Part print with two shaded views. Sizes in mm from the minimum x, y, z corner. A direction names the side the tool comes from. Round coordinates to 2 decimals unless told otherwise and drop trailing zeros. Order: outer loops, then holes, each group sorted by start corner. A loop starts at its lowest first (then second) coordinate and runs counter-clockwise, first axis right, second up. Notation, with made-up numbers: (28, 48) -> (56, 48) arc R14 cw to (56, 56) -> close; hole circle Ø9 at (-20.75, 24.25). An arc over 180 degrees is marked (long way). Use a Markdown table: item, result. Add a question column.
Item 1: Slice it at A-A, the plane z = 1.75. Give the cut face in (x, y) (3 decimals).
Item 2: 3-axis set-ups, long thin cutter, end or side, ignore diameter. For the marked faces 1, 2, 3, 4 and 5: which of +Z, -Z, +X, -X, +Y, -Y reach the whole face in a straight line?
Item 3: Slice it at C-C, the plane y = 9.5. Give the cut face in (x, z) (3 decimals), plus the area to 3 significant figures.
Item 4: Two-plate mould, pull along X, no slides. Class the marked faces 6, 7 and 8: released by +X, released by -X, zero draft, split by the parting line, or undercut.
Item 5: Probe L1, parallel to Z at x = 2.25, y = 20 (3 decimals); L2, parallel to Y at x = 8.75, z = 5 (3 decimals); L3, parallel to Y at x = 13, z = 3. List the from-to ranges inside material, lowest first.
Item 6: Slice it at D-D, the plane z = 3.75. Give the cut face in (x, y) (3 decimals).
Item 7: Pin check, flat tips, straight feed: pin 1 (1 mm diameter, centred on x = 8.5, z = 1, fed in from -Y); pin 2 (0.6 mm diameter, centred on x = 14, z = 4, fed in from +Y); pin 3 (2 mm diameter, centred on x = 5.5, y = 28.5, fed in from +Z) (3 decimals). Stop position of each tip, or through.
Item 8: Slice it at B-B, the plane x = 10.25. Give the cut face in (y, z) (3 decimals).
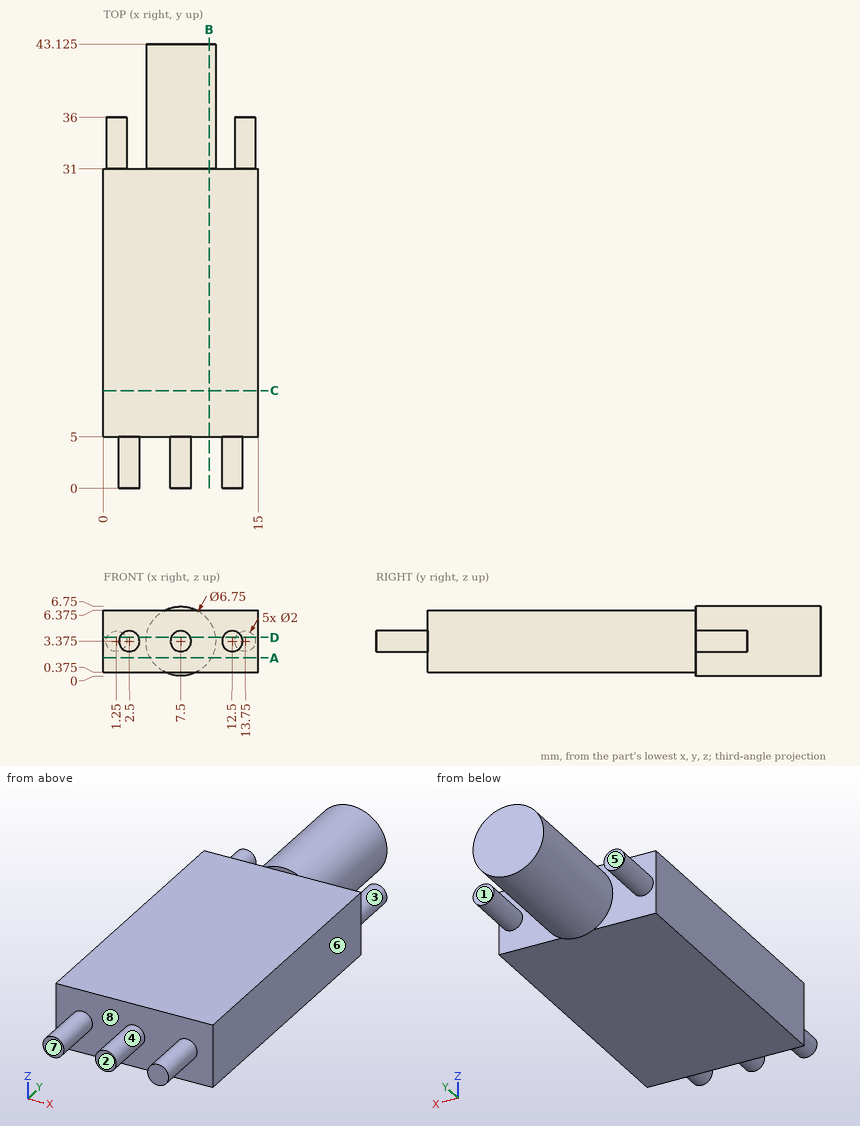
Check sheet entries:
| question | item | result |
|---|---|---|
| 1 | outline | (0, 5) -> (15, 5) -> (15, 31) -> (10.458, 31) -> (10.458, 43.125) -> (4.542, 43.125) -> (4.542, 31) -> (0, 31) -> close |
| 2 | face 1 | +Z, -Z, +X, +Y |
| 2 | face 2 | +Z, -Z, +X, -X, -Y |
| 2 | face 3 | +Y |
| 2 | face 4 | -Y |
| 2 | face 5 | +Z, -Z, -X, +Y |
| 3 | outline | (0, 0.375) -> (15, 0.375) -> (15, 6.375) -> (0, 6.375) -> close |
| 3 | area | 90.0 mm2 |
| 4 | face 6 | released by +X |
| 4 | face 7 | zero draft |
| 4 | face 8 | undercut |
| 5 | L1 | 0.375 to 6.375 |
| 5 | L2 | 5 to 43.125 |
| 5 | L3 | 0 to 36 |
| 6 | outline | (0, 5) -> (1.573, 5) -> (1.573, 0) -> (3.427, 0) -> (3.427, 5) -> (6.573, 5) -> (6.573, 0) -> (8.427, 0) -> (8.427, 5) -> (11.573, 5) -> (11.573, 0) -> (13.427, 0) -> (13.427, 5) -> (15, 5) -> (15, 31) -> (14.677, 31) -> (14.677, 36) -> (12.823, 36) -> (12.823, 31) -> (10.854, 31) -> (10.854, 43.125) -> (4.146, 43.125) -> (4.146, 31) -> (2.177, 31) -> (2.177, 36) -> (0.323, 36) -> (0.323, 31) -> (0, 31) -> close |
| 7 | pin 1 | y = 5 |
| 7 | pin 2 | y = 36 |
| 7 | pin 3 | z = 6.375 |
| 8 | outline | (5, 0.375) -> (31, 0.375) -> (31, 1.418) -> (43.125, 1.418) -> (43.125, 5.332) -> (31, 5.332) -> (31, 6.375) -> (5, 6.375) -> close |
